Could you check a few things on this model? Use its own coordinates, in mm. A direction names the side the tool comes from. Coordinates: 2 decimals unless noted, no trailing zeros. Loops run counter-clockwise (first coordinate to the right, second up) from the corner with the lowest first, then second, coordinate; pieces in that order, holes last. Notation, with made-up numbers: M 88.25,-27.5 L 129.25,-27.5 A28 cw 129.25,1.5 Z; hole C 56.5,14.5 d8. An arc over 180 degrees is marked long. Return JSON: item names as keys, results as strings. Group by question number.
from build123d import *

# Parameters (mm, degrees)
F1_DEPTH    = 2.54
F2_T1_DEPTH = 2.54
F2_T3_DEPTH = 13.5939610314
F2_T5_DEPTH = 15.8607267087
F3_T1_DEPTH = 21.0206169328
F3_T3_DEPTH = 21.2247608177


# Not quite as in the source:
# - a fillet or chamfer that OpenCascade refuses, or shapes differently, is made with other operations: its cross-section is extruded or revolved along the edge and cut away or added


with BuildPart() as f1:
    # F0 (on Front) → F1 (new body)
    with BuildSketch(Plane.XZ):
        Polygon((-31.4589329064, 0), (-36.7512629041, -5.6826620174), (-36.7512629041, -10.7626620174), (-34.308064729, -10.7626620174), (-34.308064729, -5.6826620174), (-31.4589329064, -2.6233945118), (-15.7887097448, -2.6233945118), (-13.1645070408, -6.4200807009), (-13.1645070408, -11.5000807009), (-11.3512629041, -11.5000807009), (-11.3512629041, -6.4200807009), (-15.7887097448, 0), align=None)
    extrude(amount=F1_DEPTH)

    # F2: fillet of radius 5.08 on 6 edges, made by hand

    # F2_s2 → F2_t1 (join)
    with BuildSketch(Plane.XZ):
        with BuildLine():
            ThreePointArc((-32.9656479615, -4.2412362599), (-31.2752859934, -3.0453818498), (-29.2481407001, -2.6233945118))
            Line((-29.2481407001, -2.6233945118), (-31.4589329064, -2.6233945118))
            Line((-31.4589329064, -2.6233945118), (-32.9656479615, -4.2412362599))
        make_face()
        with BuildLine():
            ThreePointArc((-18.4528550865, -2.6233945118), (-16.0934809554, -3.2045331326), (-14.2739191976, -4.8149875397))
            Line((-14.2739191976, -4.8149875397), (-15.7887097448, -2.6233945118))
            Line((-15.7887097448, -2.6233945118), (-18.4528550865, -2.6233945118))
        make_face()
        with BuildLine():
            ThreePointArc((-14.0655711519, -5.1164246759), (-13.3950022045, -6.4919857066), (-13.1645070408, -8.0048316479))
            Line((-13.1645070408, -8.0048316479), (-13.1645070408, -6.4200807009))
            Line((-13.1645070408, -6.4200807009), (-14.0655711519, -5.1164246759))
        make_face()
        with BuildLine():
            ThreePointArc((-34.308064729, -7.6818378518), (-33.9551852525, -5.8215336949), (-32.9455719904, -4.2196795999))
            Line((-32.9455719904, -4.2196795999), (-34.308064729, -5.6826620174))
            Line((-34.308064729, -5.6826620174), (-34.308064729, -7.6818378518))
        make_face()
    extrude(amount=F2_T1_DEPTH)

    # F2_s4 → F2_t3 (cut)
    with BuildSketch(Plane.XZ.offset(-5.5269805157)):
        with BuildLine():
            ThreePointArc((-32.9656479615, -1.6178417481), (-31.2752859934, -0.421987338), (-29.2481407001, 0))
            Line((-29.2481407001, 0), (-31.4589329064, 0))
            Line((-31.4589329064, 0), (-32.9656479615, -1.6178417481))
        make_face()
    extrude(amount=F2_T3_DEPTH, mode=Mode.SUBTRACT)

    # F2_s6 → F2_t5 (cut)
    with BuildSketch(Plane.XZ.offset(-6.6603633543)):
        with BuildLine():
            ThreePointArc((-18.4528550865, 0), (-16.0934809554, -0.5811386208), (-14.2739191976, -2.1915930279))
            Line((-14.2739191976, -2.1915930279), (-15.7887097448, 0))
            Line((-15.7887097448, 0), (-18.4528550865, 0))
        make_face()
    extrude(amount=F2_T5_DEPTH, mode=Mode.SUBTRACT)

    # F3: fillet of radius 5.08 on 2 edges, made by hand

    # F3_s2 → F3_t1 (cut)
    with BuildSketch(Plane.XZ.offset(-9.2403084664)):
        with BuildLine():
            ThreePointArc((-11.3512629041, -11.5000807009), (-12.6512581821, -9.8444473796), (-13.1684800157, -7.8039594497))
            Line((-13.1684800157, -7.8039594497), (-13.6760827182, -7.8240466695))
            ThreePointArc((-13.6760827182, -7.8240466695), (-13.6725070408, -8.0048316479), (-13.6725070408, -11.5000807009))
            Line((-13.6725070408, -11.5000807009), (-13.1645070408, -12.0080807009))
            ThreePointArc((-13.1645070408, -12.0080807009), (-12.2578849724, -12.0080807009), (-11.6771438954, -11.8897800459))
            Line((-11.6771438954, -11.8897800459), (-11.3512629041, -11.5000807009))
        make_face()
    extrude(amount=F3_T1_DEPTH, mode=Mode.SUBTRACT)

    # F3_s4 → F3_t3 (cut)
    with BuildSketch(Plane.XZ.offset(-9.3423804089)):
        with BuildLine():
            ThreePointArc((-34.2655455901, -7.0259517536), (-35.0733800628, -9.183691684), (-36.7512629041, -10.7626620174))
            Line((-36.7512629041, -10.7626620174), (-36.4960865494, -11.2019216536))
            ThreePointArc((-36.4960865494, -11.2019216536), (-35.5296638165, -11.2706620174), (-34.308064729, -11.2706620174))
            Line((-34.308064729, -11.2706620174), (-33.800064729, -10.7626620174))
            ThreePointArc((-33.800064729, -10.7626620174), (-33.800064729, -7.6818378518), (-33.761797504, -7.0915403635))
            Line((-33.761797504, -7.0915403635), (-34.2655455901, -7.0259517536))
        make_face()
    extrude(amount=F3_T3_DEPTH, mode=Mode.SUBTRACT)


solid = f1.part
(1) If I drill on L1, parallel to Z at x = -26.25, y = -0.75; L2, parallel to X at y = -2.4, z = -3.25; L3, parallel to X at y = -0.6, z = -4.5, over which ranges is the centre line in solid material (lowest first)? Write a range as [from, to].
(2) Imagine slicing it at A-A, the plane z = -7.25. Write out the boundary of the cut face in (x, y), then the cut area to 3 significant figures.
(3) We'd pull the mould along X, two halves only. Please class faces 1 (the face through (-24, -1, -2.623)), 2 (the face through (-16.124, -1.252, -0.565)), 3 (the face through (-36.751, -1, -8)): +X half, -X half, draft (parallel to the pull), parting line (faces both ways), or undercut.
(4) For faces 4 (the face through (-34.83, -1.25, -3.62)), 5 (the face through (-31.295, -1.252, -3.054)), which set-ups out of +Z, -Z, +X, -X, +Y, -Y let a thin tool reach every point of the face, with its end or its side?
(5) Imagine slicing it at B-B, the plane y = -1.9. Write out the boundary of the cut face in (x, z).
(6) Imagine slicing it at C-C, the plane z = -4.5. Write out the boundary of the cut face in (x, y).
(7) Imagine slicing it at D-D, the plane x = -34.75. Write out the boundary of the cut face in (y, z), then the cut area to 3 significant figures.
Checks:
{
 "1": {"L1": "[-2.62, 0]", "L2": "[-34.49, -31.69], [-16.01, -13.54]", "L3": "[-35.65, -33.19], [-14.51, -12.68]"},
 "2": {"outline": "M -36.75,-2.54 L -34.3,-2.54 L -34.3,0 L -36.75,0 Z; M -13.22,-2.54 L -11.35,-2.54 L -11.35,0 L -13.22,0 Z", "area": "11.0 mm²"},
 "3": {"face 1": "undercut", "face 2": "+X half", "face 3": "-X half"},
 "4": {"face 4": "+Z, -X, +Y, -Y", "face 5": "-Z, +Y, -Y"},
 "5": {"outline": "M -36.75,-10.76 A5.08 ccw -34.27,-7.03 A5.08 cw -32.96,-4.23 A5.08 cw -29.25,-2.62 L -18.45,-2.62 A5.08 cw -14.27,-4.81 L -14.07,-5.12 A5.08 cw -13.17,-7.8 A5.08 ccw -11.35,-11.5 L -11.35,-6.42 L -14.27,-2.19 A5.08 ccw -18.45,0 L -29.25,0 A5.08 ccw -32.97,-1.62 L -36.75,-5.68 Z"},
 "6": {"outline": "M -35.65,-2.54 L -33.19,-2.54 L -33.19,0 L -35.65,0 Z; M -14.51,-2.54 L -12.68,-2.54 L -12.68,0 L -14.51,0 Z"},
 "7": {"outline": "M -2.54,-8.62 L 0,-8.62 L 0,-3.53 L -2.54,-3.53 Z", "area": "12.9 mm²"}
}
